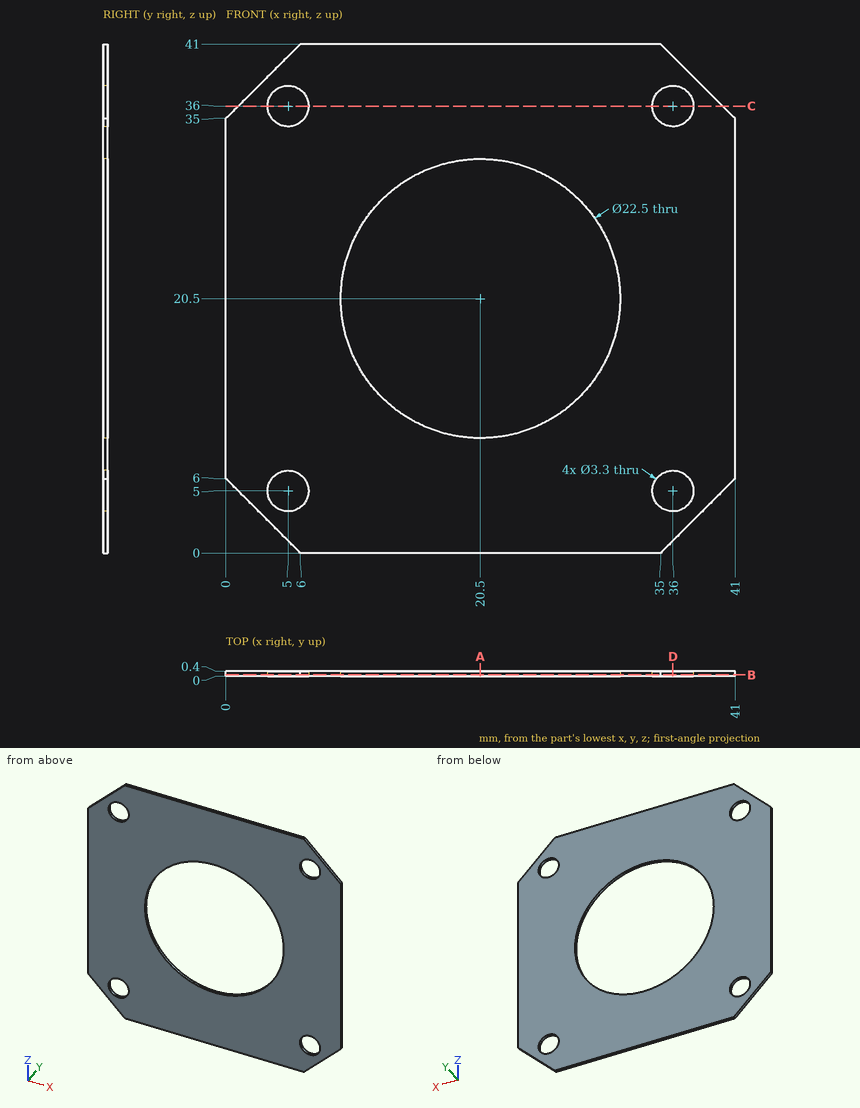
The figure shows three views and two pictorial views of one solid part (mm, origin at its lowest corner). Answer the questions. Give positions to 0.01 mm unless a question says otherwise; leave off trailing zeros. Loops run counter-clockwise (first coordinate to the right, second up) from the corner with the lowest first, then second, coordinate; pieces in that order, holes last. Notation, with made-up numbers: (-7, 3.25) - (47, 3.25) arc R23 cw to (47, 37.25) - close; hole circle Ø11 at (-3.5, -25). An arc over 180 degrees is marked (long way). Answer in a Markdown table with one row per item.
(1) Section D-D (x = 36) is taken. Give the vertices of the cut face in (y, z).
Results list:
| item | result |
|---|---|
| outline | (0, 1) - (0.4, 1) - (0.4, 3.35) - (0, 3.35) - close; (0, 6.65) - (0.4, 6.65) - (0.4, 34.35) - (0, 34.35) - close; (0, 37.65) - (0.4, 37.65) - (0.4, 40) - (0, 40) - close |
(2) A flat-ended cylindrical pin translates along its axis: pin 1 Ø2 at (x, z) = (36, 5) entering from -Y. Find the tip coordinate at first contact, or state that the pin passes through.
Results list:
| item | result |
|---|---|
| pin 1 | passes through |
(3) Section A-A (x = 20.5) is taken. Give the vertices of the cut face in (y, z).
Results list:
| item | result |
|---|---|
| outline | (0, 0) - (0.4, 0) - (0.4, 9.25) - (0, 9.25) - close; (0, 31.75) - (0.4, 31.75) - (0.4, 41) - (0, 41) - close |
(4) Section C-C (z = 36) is taken. Give the vertices of the cut face in (x, y), and give its area (3 significant figures).
Results list:
| item | result |
|---|---|
| outline | (1, 0) - (3.35, 0) - (3.35, 0.4) - (1, 0.4) - close; (6.65, 0) - (34.35, 0) - (34.35, 0.4) - (6.65, 0.4) - close; (37.65, 0) - (40, 0) - (40, 0.4) - (37.65, 0.4) - close |
| area | 13.0 mm² |
(5) Section B-B (y = 0.1) is taken. Give the vertices of the cut face in (x, z).
Results list:
| item | result |
|---|---|
| outline | (0, 6) - (6, 0) - (35, 0) - (41, 6) - (41, 35) - (35, 41) - (6, 41) - (0, 35) - close; hole circle Ø3.3 at (5, 5); hole circle Ø3.3 at (5, 36); hole circle Ø22.5 at (20.5, 20.5); hole circle Ø3.3 at (36, 5); hole circle Ø3.3 at (36, 36) |
(6) Consider L1, parallel to Z at x = 20.5, y = 0.2; L2, parallel to Z at x = 36, y = 0.15; L3, parallel to Z at x = 36.5, y = 0.3. Determine where each line is inside the solid, lowest interval first. Write a range as [from, to].
Results list:
| item | result |
|---|---|
| L1 | z = [0, 9.25], [31.75, 41] |
| L2 | z = [1, 3.35], [6.65, 34.35], [37.65, 40] |
| L3 | z = [1.5, 3.43], [6.57, 34.43], [37.57, 39.5] |
